Source: CAD feature listing. Evaluate the final solid. Frame: model axes, mm. Round coordinates to 2 decimals unless told otherwise and drop trailing zeros. Loops run counter-clockwise (first coordinate to the right, second up) from the corner with the lowest first, then second, coordinate; pieces in that order, holes last. Notation, with made-up numbers: M 67.25,64 L 73.25,64 A9 ccw 73.25,78 Z; hole C 7,8 d2. An arc over 180 degrees is marked long. Answer as a JSON object with one key per item and string values.
from build123d import *

# Parameters (mm, degrees)
SKETCH1_W           = 200
SKETCH1_H           = 90
BOSS_EXTRUDE1_DEPTH = 3
SKETCH2_R           = 2.5
CUT_EXTRUDE1_DEPTH  = 4
SKETCH3_R           = 1.016
CUT_EXTRUDE2_DEPTH  = 4


with BuildPart() as part:
    # Sketch1 → Boss-Extrude1 (new body)
    with BuildSketch(Plane(origin=(0, 0, 0), x_dir=(1, 0, 0), z_dir=(0, 1, 0))):
        Rectangle(SKETCH1_W, SKETCH1_H)
    extrude(amount=BOSS_EXTRUDE1_DEPTH)

    # Sketch2 → Cut-Extrude1 (cut, through all)
    with BuildSketch(Plane(origin=(0, 3, 0), x_dir=(1, 0, 0), z_dir=(0, 1, 0))):
        with Locations((-77.5, 40)):
            Circle(SKETCH2_R)
        with Locations((77.5, 40)):
            Circle(SKETCH2_R)
        with Locations((77.5, -40)):
            Circle(SKETCH2_R)
        with Locations((-77.5, -40)):
            Circle(SKETCH2_R)
    extrude(amount=-CUT_EXTRUDE1_DEPTH, mode=Mode.SUBTRACT)

    # Sketch3 → Cut-Extrude2 (cut, through all)
    with BuildSketch(Plane(origin=(0, 3, 0), x_dir=(1, 0, 0), z_dir=(0, 1, 0))):
        with Locations((-44.45, 22.098)):
            Circle(SKETCH3_R)
        with Locations((-44.45, -22.098)):
            Circle(SKETCH3_R)
        with Locations((35.56, 0)):
            Circle(SKETCH3_R)
    extrude(amount=-CUT_EXTRUDE2_DEPTH, mode=Mode.SUBTRACT)


solid = part.part
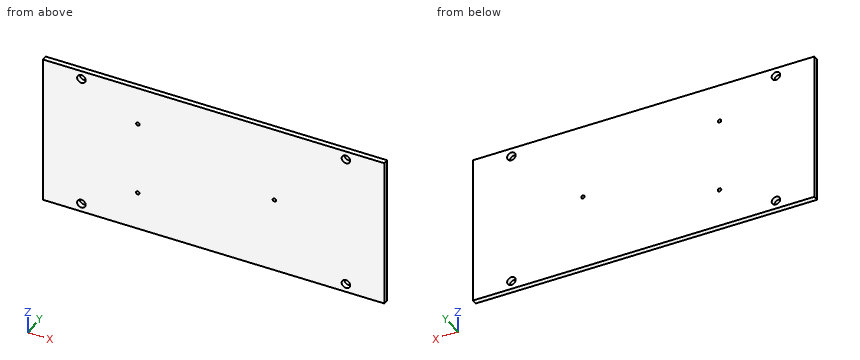
Item 1: Section A-A on z = -40. Return the cut outline in (x, y).
Answer sheet:
{"outline": "M -100,0 L -80,0 L -80,3 L -100,3 Z; M -75,0 L 75,0 L 75,3 L -75,3 Z; M 80,0 L 100,0 L 100,3 L 80,3 Z"}
Item 2: Section B-B on x = 77.5. Return the cut outline in (y, z), then the cut area to 3 significant figures.
Answer sheet:
{"outline": "M 0,-45 L 3,-45 L 3,-42.5 L 0,-42.5 Z; M 0,-37.5 L 3,-37.5 L 3,37.5 L 0,37.5 Z; M 0,42.5 L 3,42.5 L 3,45 L 0,45 Z", "area": "240 mm²"}
Item 3: Line query: probe 1 along X at (y, z) = (1.2, 40); probe 2 along Z at (x, y) = (-77.5, 0.85); probe 3 along X at (y, z) = (1.15, -39). Output: solid intervals per line, ascending. Write a range as from..to.
Answer sheet:
{"probe 1": "x = -100..-80, -75..75, 80..100", "probe 2": "z = -45..-42.5, -37.5..37.5, 42.5..45", "probe 3": "x = -100..-79.79, -75.21..75.21, 79.79..100"}
